Read the model definition and answer for the solid it produces. Units are mm, in the model's axes. Coordinates: 2 decimals unless noted, no trailing zeros. Loops run counter-clockwise (first coordinate to the right, second up) from the corner with the lowest first, then second, coordinate; pieces in that order, holes last. Notation, with made-up numbers: (74, -3.5) -> (88, -3.5) arc R17 ccw to (88, 5.5) -> close; hole circle Ø11 at (68.25, 27). An arc over 180 degrees is marked (long way). Answer as a JSON object with one key per item and string values. Group by question number.
Q1. The part is cut by section B-B on y = 32.5. Write down the section's boundary in (x, z).
Q2. The part is cut by section A-A on z = 0. Write down the section's boundary in (x, y).
Q3. The part is cut by section D-D on y = -3.5. Write down the section's boundary in (x, z).
Q4. The part is cut by section C-C on x = 1.2. State how many separate pieces and enclosed holes the cut face has, and give its area (3 significant figures).
Q5. Straight lines are drawn through the part: line 1 along Y through (x, z) = (1.65, -0.5); line 2 along Z through (x, y) = (2.3, 43.5); line 3 along Y through (x, z) = (2.65, 2). For each, find the intervals that lie inside material, in ascending order. Write a range as [from, to].
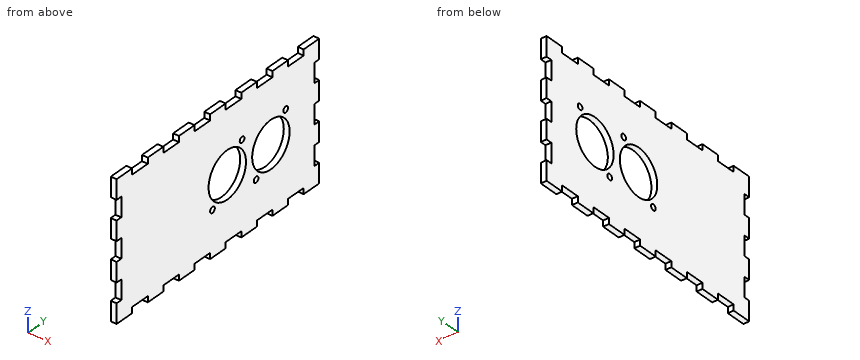
from build123d import *

# Parameters (mm, degrees)
F0_W     = 130
F0_H     = 70
F1_DEPTH = 3
F2_W     = 3
F2_H     = 10
F2_W_2   = 10
F2_H_2   = 3
F3_DEPTH = 3.001
F4_R     = 12
F4_R_2   = 1.5
F5_DEPTH = 3.001


with BuildPart() as f1:
    # F0 (on Right) → F1 (new body)
    with BuildSketch(Plane.YZ):
        Rectangle(F0_W, F0_H)
    extrude(amount=F1_DEPTH)

    # F2 (on face) → F3 (cut, through all)
    with BuildSketch(Plane.YZ.offset(3)):
        with Locations((-63.5, 20)):
            Rectangle(F2_W, F2_H)
        with Locations((-63.5, 0)):
            Rectangle(F2_W, F2_H)
        with Locations((-63.5, -20)):
            Rectangle(F2_W, F2_H)
        with Locations((63.5, 0)):
            Rectangle(F2_W, F2_H)
        with Locations((63.5, 20)):
            Rectangle(F2_W, F2_H)
        with Locations((63.5, -20)):
            Rectangle(F2_W, F2_H)
        with Locations((-50, -33.5)):
            Rectangle(F2_W_2, F2_H_2)
        with Locations((-30, -33.5)):
            Rectangle(F2_W_2, F2_H_2)
        with Locations((-10, -33.5)):
            Rectangle(F2_W_2, F2_H_2)
        with Locations((10, -33.5)):
            Rectangle(F2_W_2, F2_H_2)
        with Locations((30, -33.5)):
            Rectangle(F2_W_2, F2_H_2)
        with Locations((50, -33.5)):
            Rectangle(F2_W_2, F2_H_2)
        with Locations((-50, 33.5)):
            Rectangle(F2_W_2, F2_H_2)
        with Locations((-30, 33.5)):
            Rectangle(F2_W_2, F2_H_2)
        with Locations((50, 33.5)):
            Rectangle(F2_W_2, F2_H_2)
        with Locations((-10, 33.5)):
            Rectangle(F2_W_2, F2_H_2)
        with Locations((10, 33.5)):
            Rectangle(F2_W_2, F2_H_2)
        with Locations((30, 33.5)):
            Rectangle(F2_W_2, F2_H_2)
    extrude(amount=-F3_DEPTH, mode=Mode.SUBTRACT)

    # F4 (on face) → F5 (cut, through all)
    with BuildSketch(Plane.YZ.offset(3)):
        with Locations((34, 0)):
            Circle(F4_R)
        with Locations((43.5, 12)):
            Circle(F4_R_2)
        with Locations((24.5, -12)):
            Circle(F4_R_2)
        with Locations((6, 0)):
            Circle(F4_R)
        with Locations((-3.5, -12)):
            Circle(F4_R_2)
        with Locations((15.5, 12)):
            Circle(F4_R_2)
    extrude(amount=-F5_DEPTH, mode=Mode.SUBTRACT)


solid = f1.part
Final values:
{
 "1": {"outline": "(0, -32) -> (3, -32) -> (3, -11.91) -> (0, -11.91) -> close; (0, 11.91) -> (3, 11.91) -> (3, 32) -> (0, 32) -> close"},
 "2": {"outline": "(0, -62) -> (3, -62) -> (3, -6) -> (0, -6) -> close; (0, 18) -> (3, 18) -> (3, 22) -> (0, 22) -> close; (0, 46) -> (3, 46) -> (3, 62) -> (0, 62) -> close"},
 "3": {"outline": "(0, -35) -> (3, -35) -> (3, -13.5) -> (0, -13.5) -> close; (0, -10.5) -> (3, -10.5) -> (3, -7.33) -> (0, -7.33) -> close; (0, 7.33) -> (3, 7.33) -> (3, 35) -> (0, 35) -> close"},
 "4": {"separate pieces": "1", "enclosed holes": "6", "area": "7,630 mm2"},
 "5": {"line 1": "y = [-62, -5.99], [17.99, 22.01], [45.99, 62]", "line 2": "z = [-35, -7.33], [7.33, 10.5], [13.5, 35]", "line 3": "y = [-62, -5.83], [17.83, 22.17], [45.83, 62]"}
}
